```python
from build123d import *

# Parameters (mm, degrees)
SKETCH1_W           = 111
SKETCH1_H           = 30.5
BOSS_EXTRUDE1_DEPTH = 2
SKETCH2_W           = 111
SKETCH2_H           = 30.5
SKETCH2_W_2         = 107
SKETCH2_H_2         = 26.5
BOSS_EXTRUDE2_DEPTH = 19
FILLET1_R           = 2
SKETCH4_R           = 2
BOSS_EXTRUDE4_DEPTH = 3
SKETCH5_R           = 1.75
SKETCH5_R_2         = 0.75
BOSS_EXTRUDE5_DEPTH = 6.4
SKETCH6_W           = 8.3
SKETCH6_H           = 6
CUT_EXTRUDE1_DEPTH  = 2
FILLET2_R           = 1
SKETCH7_R           = 0.75
CUT_EXTRUDE3_DEPTH  = 2.5
FILLET3_R           = 1


with BuildPart() as part:
    # Sketch1 → Boss-Extrude1 (new body)
    with BuildSketch(Plane(origin=(0, 0, 0), x_dir=(1, 0, 0), z_dir=(0, 1, 0))):
        with Locations((55.5, 15.25)):
            Rectangle(SKETCH1_W, SKETCH1_H)
    extrude(amount=BOSS_EXTRUDE1_DEPTH)

    # Sketch2 → Boss-Extrude2 (add)
    with BuildSketch(Plane(origin=(0, 2, 0), x_dir=(1, 0, 0), z_dir=(0, 1, 0))):
        with Locations((55.5, 15.25)):
            Rectangle(SKETCH2_W, SKETCH2_H)
        with Locations((55.5, 15.25)):
            Rectangle(SKETCH2_W_2, SKETCH2_H_2, mode=Mode.SUBTRACT)
    extrude(amount=BOSS_EXTRUDE2_DEPTH)

    # Fillet1
    fillet1_edges = [part.edges().sort_by_distance(p)[0] for p in [
        (55.5, 0, -30.5),
        (111, 0, -15.25),
        (55.5, 0, 0),
        (0, 0, -15.25),
        (0, 10.5, -30.5),
        (111, 10.5, -30.5),
        (111, 10.5, 0),
        (0, 10.5, 0),
    ]]
    fillet(fillet1_edges, radius=FILLET1_R)

    # Sketch4 → Boss-Extrude4 (add)
    with BuildSketch(Plane(origin=(0, 21, 0), x_dir=(1, 0, 0), z_dir=(0, 1, 0))):
        with Locations((2, 28.5)):
            Circle(SKETCH4_R)
        with Locations((2, 2)):
            Circle(SKETCH4_R)
        with Locations((109, 2)):
            Circle(SKETCH4_R)
        with Locations((109, 28.5)):
            Circle(SKETCH4_R)
    extrude(amount=-BOSS_EXTRUDE4_DEPTH)

    # Sketch5 → Boss-Extrude5 (add)
    with BuildSketch(Plane(origin=(0, 2, 0), x_dir=(1, 0, 0), z_dir=(0, 1, 0))):
        with Locations((63.39, 23.825)):
            Circle(SKETCH5_R)
        with Locations((63.39, 23.825)):
            Circle(SKETCH5_R_2, mode=Mode.SUBTRACT)
        with Locations((63.39, 6.675)):
            Circle(SKETCH5_R)
        with Locations((63.39, 6.675)):
            Circle(SKETCH5_R_2, mode=Mode.SUBTRACT)
        with Locations((78, 6.675)):
            Circle(SKETCH5_R)
        with Locations((78, 6.675)):
            Circle(SKETCH5_R_2, mode=Mode.SUBTRACT)
        with Locations((78, 23.825)):
            Circle(SKETCH5_R)
        with Locations((78, 23.825)):
            Circle(SKETCH5_R_2, mode=Mode.SUBTRACT)
    extrude(amount=BOSS_EXTRUDE5_DEPTH)

    # Sketch6 → Cut-Extrude1 (cut)
    with BuildSketch(Plane.XY):
        with Locations((54.88, 11.4)):
            Rectangle(SKETCH6_W, SKETCH6_H)
    extrude(amount=-CUT_EXTRUDE1_DEPTH, mode=Mode.SUBTRACT)

    # Fillet2
    fillet2_edges = [part.edges().sort_by_distance(p)[0] for p in [
        (59.03, 8.4, -1),
        (59.03, 14.4, -1),
        (50.73, 14.4, -1),
        (50.73, 8.4, -1),
    ]]
    fillet(fillet2_edges, radius=FILLET2_R)

    # Sketch7 → Cut-Extrude3 (cut)
    with BuildSketch(Plane(origin=(0, 21, 0), x_dir=(1, 0, 0), z_dir=(0, 1, 0))):
        with Locations((2, 28.5)):
            Circle(SKETCH7_R)
        with Locations((2, 2)):
            Circle(SKETCH7_R)
        with Locations((109, 2)):
            Circle(SKETCH7_R)
        with Locations((109, 28.5)):
            Circle(SKETCH7_R)
    extrude(amount=-CUT_EXTRUDE3_DEPTH, mode=Mode.SUBTRACT)

    # Fillet3
    fillet3_edges = [part.edges().sort_by_distance(p)[0] for p in [
        (54.88, 14.4, 0),
        (59.03, 11.4, 0),
        (50.73, 11.4, 0),
        (54.88, 8.4, 0),
        (58.737106781, 14.107106781, 0),
        (51.022893219, 14.107106781, 0),
        (51.022893219, 8.692893219, 0),
        (58.737106781, 8.692893219, 0),
    ]]
    fillet(fillet3_edges, radius=FILLET3_R)


solid = part.part
```
The listing builds one solid part. Answer for the finished solid, in the listing's coordinates (mm). A direction names the side the tool comes from. Round coordinates to 2 decimals unless told otherwise and drop trailing zeros. Write each loop counter-clockwise with the first axis right and the second up, starting at its lowest first coordinate (ties: lowest second). Pieces come first, ordered by that corner, then holes. Notation, with made-up numbers: (16, 44) -> (55, 44) arc R28 ccw to (55, 81) -> close; hole circle Ø3 at (52, 4.5). An arc over 180 degrees is marked (long way). Use CSV: the item, a comma, the result in double quotes. Start each with the question number.
(1) The mould has two halves that part along Y. Classify faces 4 (the face through (108, 18, -3)), 5 (the face through (43, 21, -29)), 6 (the face through (107.6, 19.52, -3.43)): released by +Y, released by -Y, zero draft, split by the parting line, or undercut.
(2) Section C-C on z = -10 is taken. Give the vertices of the cut face in (x, y), then the cut area to 3 significant figures.
(3) Section A-A on y = 19.5 is taken. Give the vertices of the cut face in (x, z), then the cut area to 3 significant figures.
(4) Consider L1, parallel to Z at x = 63.39, y = 4.5 (3 decimals); L2, parallel to Z at x = 31, y = 12.25; L3, parallel to X at y = 8.5, z = -11. Determine where each line is inside the solid, lowest interval first. Write a range as from..to.
(5) Section B-B on x = 55 is taken. Give the vertices of the cut face in (y, z).
(6) Section D-D on x = 9 is taken. Give the vertices of the cut face in (y, z), then the cut area to 3 significant figures.
(7) Which of the six approach directions +Z, -Z, +X, -X, +Y, -Y give full straight-line access (tool end or side, diameter ignored) to faces 1 (the face through (55, 7, 0)), 2 (the face through (79.67, 5.16, -7.2)), 3 (the face through (108, 18, -28))?
(8) Each of these flat-tipped pins is pushed along its axis until it touches: pin 1 (1.6 mm diameter, centred on x = 2, z = -28.5, fed in from +Y); pin 2 (0.8 mm diameter, centred on x = 78, z = -24, fed in from +Y); pin 3 (1.8 mm diameter, centred on x = 77.5, z = -7, fed in from +Y). Where does it stop, or does it pass through?
A:
1,face 4,"undercut"
1,face 5,"released by +Y"
1,face 6,"zero draft"
2,outline,"(0, 2) arc R2 ccw to (2, 0) -> (109, 0) arc R2 ccw to (111, 2) -> (111, 21) -> (109, 21) -> (109, 2) -> (2, 2) -> (2, 21) -> (0, 21) -> close"
2,area,"296 mm²"
3,outline,"(0, -28.5) arc R2 ccw to (2, -30.5) -> (109, -30.5) arc R2 ccw to (111, -28.5) -> (111, -2) arc R2 ccw to (109, 0) -> (2, 0) arc R2 ccw to (0, -2) -> close; hole circle Ø1.5 at (2, -28.5); hole circle Ø1.5 at (2, -2); hole (2, -26.5) arc R2 cw to (4, -28.5) -> (107, -28.5) arc R2 cw to (109, -26.5) -> (109, -4) arc R2 cw to (107, -2) -> (4, -2) arc R2 cw to (2, -4) -> close; hole circle Ø1.5 at (109, -28.5); hole circle Ø1.5 at (109, -2)"
3,area,"552 mm²"
4,L1,"z = -30.5..-28.5, -25.575..-24.575, -23.075..-22.075, -8.425..-7.425, -5.925..-4.925, -2..0"
4,L2,"z = -30.5..-28.5, -2..0"
4,L3,"x = 0..2, 109..111"
5,outline,"(0, -28.5) arc R2 ccw to (2, -30.5) -> (21, -30.5) -> (21, -28.5) -> (2, -28.5) -> (2, -2) -> (8.4, -2) -> (8.4, -1) arc R1 ccw to (7.4, 0) -> (2, 0) arc R2 ccw to (0, -2) -> close; (14.4, -2) -> (21, -2) -> (21, 0) -> (15.4, 0) arc R1 ccw to (14.4, -1) -> close"
6,outline,"(0, -28.5) arc R2 ccw to (2, -30.5) -> (21, -30.5) -> (21, -28.5) -> (2, -28.5) -> (2, -2) -> (21, -2) -> (21, 0) -> (2, 0) arc R2 ccw to (0, -2) -> close"
6,area,"135 mm²"
7,face 1,"+Z, +X, -X, +Y, -Y"
7,face 2,"+Y"
7,face 3,"none"
8,pin 1,"stops at y = 21"
8,pin 2,"stops at y = 2"
8,pin 3,"stops at y = 8.4"
